For this review, take the finished solid that the model builds, in its own axes (mm). Round coordinates to 2 decimals unless told otherwise and drop trailing zeros. Write each loop counter-clockwise with the first axis right and the second up, starting at its lowest first coordinate (ties: lowest second). Pieces come first, ordered by that corner, then holes. Notation, with made-up numbers: M -16,-29.5 L -6,-29.5 A34 cw -6,2.5 Z; hole C -7.5,-25 d6. An arc over 180 degrees is marked long. Use one line per item in the form item = value. Start each with the question number.
Item 1: For P1, Ø8, axis at y = 18, z = 8.5, coming from the +X side; P2, Ø2, axis at x = 19.5, y = 119.5, coming from the +Z side; P3, Ø4, axis at y = 105, z = 34, coming from the -X side, all flat-tipped, find the tip position at first contact; note any pin that passes through.
Item 2: Add section C-C (x = 21). State the section outline as (y, z) points.
Item 3: Draft analysis for pull direction Y (two halves, no side actions). For faces 1 (the flat face through (12.7, 119, 24)), 2 (the flat face through (0, 114, 19)), 3 (the flat face through (12.7, 11, 19)), 4 (the cylindrical face through (34.28, 3.62, 18.96)), state which applies: released by +Y, released by -Y, zero draft, split by the parting line, or undercut.
Item 4: Add section B-B (x = 6). State the section outline as (y, z) points, and give its area (3 significant figures).
Item 5: For line 1 (Y direction, x = 19, z = 19); line 2 (Y direction, x = 4, z = 17.5); line 3 (Z direction, x = 26, y = 101.5), list the stretches that pass through material, from the lowest coordinate up. Write a range as [from, to].
Item 6: Add section A-A (y = 58.5). State the section outline as (x, z) points, and give its area (3 significant figures).
from build123d import *

# Parameters (mm, degrees)
F1_DEPTH = 38.1
F2_R     = 12.7
F4_DEPTH = 12.7


with BuildPart() as f1:
    # F0 (on Right) → F1 (new body)
    with BuildSketch(Plane.YZ):
        with BuildLine():
            ThreePointArc((0, 12.7), (3.7197438789, 3.7197438789), (12.7, 0))
            Line((12.7, 0), (88.9, 0))
            Line((88.9, 0), (114.3, 0))
            ThreePointArc((114.3, 0), (133.35, 19.05), (114.3, 38.1))
            Line((114.3, 38.1), (88.9, 38.1))
            Line((88.9, 38.1), (12.7, 38.1))
            ThreePointArc((12.7, 38.1), (3.7197438789, 34.3802561211), (0, 25.4))
            Line((0, 25.4), (0, 12.7))
        make_face()
    extrude(amount=F1_DEPTH)

    # F2
    f2_edges = [f1.edges().sort_by_distance(p)[0] for p in [
        (38.1, 0, 19.05),
        (38.1, 3.719744, 3.719744),
        (38.1, 63.5, 0),
        (38.1, 133.35, 19.05),
        (38.1, 63.5, 38.1),
        (38.1, 3.719744, 34.380256),
        (0, 0, 19.05),
        (0, 3.719744, 3.719744),
        (0, 63.5, 0),
        (0, 133.35, 19.05),
        (0, 63.5, 38.1),
        (0, 3.719744, 34.380256),
    ]]
    fillet(f2_edges, radius=F2_R)

    # F3 (on face) → F4 (cut)
    with BuildSketch(Plane(origin=(0, 0, 0), x_dir=(0, -1, 0), z_dir=(-1, 0, 0))):
        with BuildLine():
            ThreePointArc((-114.3, 25.4), (-109.8098719395, 23.5401280605), (-107.95, 19.05))
            ThreePointArc((-107.95, 19.05), (-109.8098719395, 14.5598719395), (-114.3, 12.7))
            Line((-114.3, 12.7), (-96.3394877579, 12.7))
            ThreePointArc((-96.3394877579, 12.7), (-95.5243474386, 15.8286073053), (-95.25, 19.05))
            ThreePointArc((-95.25, 19.05), (-95.5243474386, 22.2713926947), (-96.3394877579, 25.4))
            Line((-96.3394877579, 25.4), (-114.3, 25.4))
        make_face()
        with BuildLine():
            ThreePointArc((-114.3, 12.7), (-120.65, 19.05), (-114.3, 25.4))
            Line((-114.3, 25.4), (-96.3394877579, 25.4))
            ThreePointArc((-96.3394877579, 25.4), (-133.35, 19.05), (-96.3394877579, 12.7))
            Line((-96.3394877579, 12.7), (-114.3, 12.7))
        make_face()
        with BuildLine():
            Line((-19.05, 25.4), (-37.0105122421, 25.4))
            ThreePointArc((-37.0105122421, 25.4), (-38.1, 19.05), (-37.0105122421, 12.7))
            Line((-37.0105122421, 12.7), (-19.0500000394, 12.7))
            ThreePointArc((-19.0500000394, 12.7), (-25.4, 19.0500000197), (-19.05, 25.4))
        make_face()
        with BuildLine():
            ThreePointArc((-19.3726803674, 38.0972669268), (-30.1798665694, 34.5105488307), (-37.0105122421, 25.4))
            Line((-37.0105122421, 25.4), (-19.05, 25.4))
            Line((-19.05, 25.4), (-12.7, 25.4))
            Line((-12.7, 25.4), (-12.7, 19.05))
            Line((-12.7, 19.05), (-12.7, 12.7))
            Line((-12.7, 12.7), (-19.0500000394, 12.7))
            Line((-19.0500000394, 12.7), (-37.0105122421, 12.7))
            ThreePointArc((-37.0105122421, 12.7), (-30.0485226281, 3.4957401333), (-19.05, 0))
            Line((-19.05, 0), (-15.2826001868, -14.698324725))
            Line((-15.2826001868, -14.698324725), (7.5956550427, -14.698324725))
            Line((7.5956550427, -14.698324725), (22.0383554697, 45.6287078559))
            Line((22.0383554697, 45.6287078559), (-15.4104121029, 51.7636574805))
            Line((-15.4104121029, 51.7636574805), (-19.3726803674, 38.0972669268))
        make_face()
        with BuildLine():
            Line((-12.7, 25.4), (-19.05, 25.4))
            ThreePointArc((-19.05, 25.4), (-14.5598719395, 23.5401280605), (-12.7, 19.05))
            Line((-12.7, 19.05), (-12.7, 25.4))
        make_face()
        with BuildLine():
            ThreePointArc((-12.7, 19.05), (-14.5598719534, 14.5598719255), (-19.0500000394, 12.7))
            Line((-19.0500000394, 12.7), (-12.7, 12.7))
            Line((-12.7, 12.7), (-12.7, 19.05))
        make_face()
    extrude(amount=-F4_DEPTH, mode=Mode.SUBTRACT)


solid = f1.part
Calculated:
q1.P1 = 38.1
q1.P2 = 37.63
q1.P3 = 3.76
q2.outline = M 0,12.7 A12.7 ccw 12.7,0 L 114.3,0 A19.05 ccw 114.3,38.1 L 12.7,38.1 A12.7 ccw 0,25.4 Z
q3.face_1 = undercut
q3.face_2 = zero draft
q3.face_3 = undercut
q3.face_4 = released by -Y
q4.outline = C 19.05,19.05 d12.7; M 27.37,1.91 L 105.98,1.91 A19.05 cw 105.98,36.19 L 27.37,36.19 A19.05 cw Z; C 114.3,19.05 d12.7
q4.area = 2,420 mm^2
q5.line_1 = [0, 133.35]
q5.line_2 = [12.89, 25.21], [38.04, 95.31], [108.14, 120.46]
q5.line_3 = [0.01, 38.09]
q6.outline = M 0,12.7 A12.7 ccw 12.7,0 L 25.4,0 A12.7 ccw 38.1,12.7 L 38.1,25.4 A12.7 ccw 25.4,38.1 L 12.7,38.1 A12.7 ccw 0,25.4 Z
q6.area = 1,310 mm^2
